Answer from the drawing. Dimensions are ordinates in mm from the lowest x, y and z of the part. A direction names the side the tool comes from. Give positions to 0.01 mm unless a question says otherwise; leave off trailing zeros. Loops run counter-clockwise (first coordinate to the right, second up) from the corner with the lowest first, then second, coordinate; pieces in that order, holes last. Notation, with made-up numbers: (-25.75, 61.5) - (-0.75, 61.5) arc R14 cw to (-0.75, 78.5) - close; hole circle Ø10 at (7, 29.5). An arc over 180 degrees is marked (long way). One line per item, written item: value.
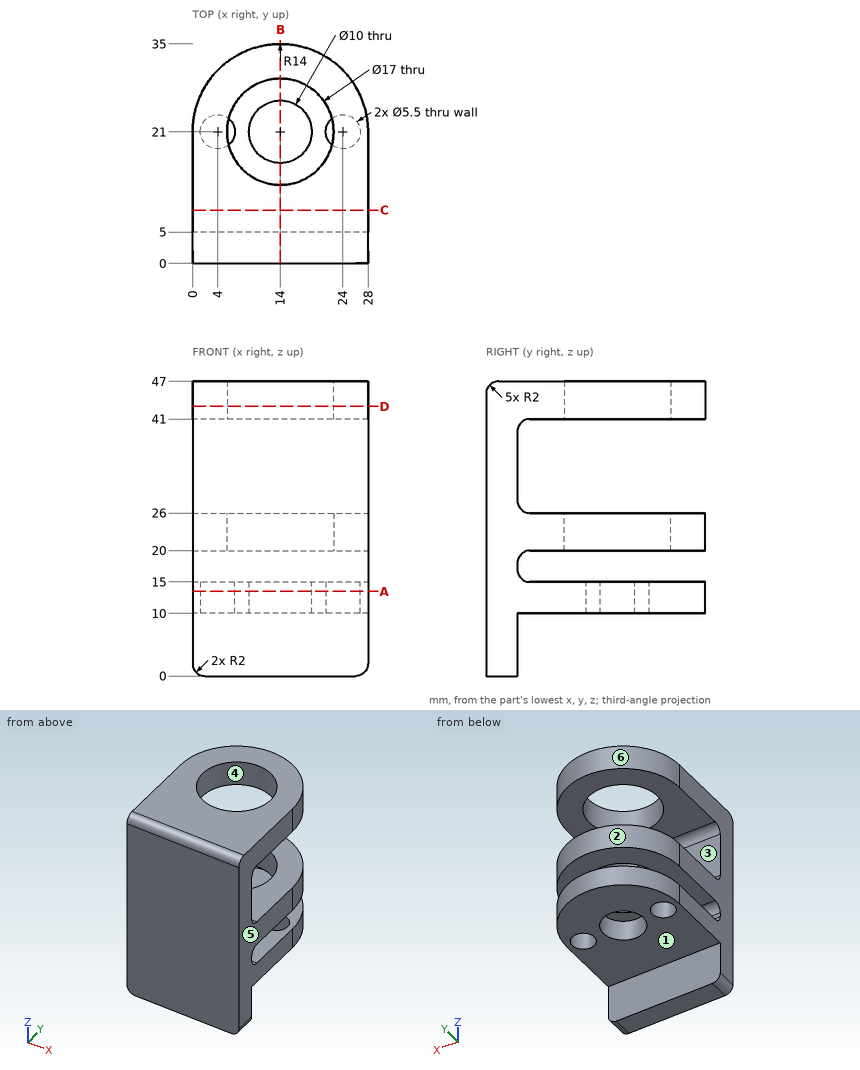
1. Section A-A (z = 13.5) is taken. Write down the section's boundary in (x, y).
Output:
outline: (0, 0) - (28, 0) - (28, 21) arc R14 ccw to (0, 21) - close; hole circle Ø5.5 at (4, 21); hole circle Ø10 at (14, 21); hole circle Ø5.5 at (24, 21)
2. Find the intervals of material crossed by line 1 along Z through (x, y) = (3, 13); line 2 along Y through (x, z) = (14, 22.6); line 3 along Y through (x, z) = (23.75, 37), in increasing order.
Output:
line 1: z = 10 to 15, 20 to 26, 41 to 47
line 2: y = 0 to 12.5, 29.5 to 35
line 3: y = 0 to 5
3. Section C-C (y = 8.5) is taken. Write down the section's boundary in (x, z).
Output:
outline: (0, 10) - (28, 10) - (28, 15) - (0, 15) - close; (0, 20) - (28, 20) - (28, 26) - (0, 26) - close; (0, 41) - (28, 41) - (28, 47) - (0, 47) - close
4. The mould has two halves that part along X. Classify the marked faces 4, 5 and 6: released by +X, released by -X, zero draft, split by the parting line, or undercut.
Output:
face 4: undercut
face 5: released by +X
face 6: split by the parting line
5. Flat-ended cylindrical pins translate along their axes: pin 1 Ø2 at (x, z) = (19, 35.5) entering from -Y; pin 2 Ø4 at (x, y) = (19.5, 22) entering from +Z; pin 3 Ø5 at (x, z) = (12.5, 5.5) entering from +Y; pin 4 Ø8.5 at (x, y) = (18.5, 21.5) entering from -Z. Find the tip coordinate at first contact, or state that the pin passes through.
Output:
pin 1: stops at y = 0
pin 2: stops at z = 15
pin 3: stops at y = 5
pin 4: stops at z = 10
6. Section B-B (x = 14) is taken. Count the separate pieces of the cut face and the enclosed holes in it, and give its area (3 significant figures).
Output:
separate pieces: 4
enclosed holes: 0
area: 494 mm²
7. For the marked faces 1, 2 and 3, determine the directions among +Z, -Z, +X, -X, +Y, -Y from which every point of the face is accessible in a straight line to the end or side of a thin tool.
Output:
face 1: -Z, +X, -X, +Y
face 2: +Z, -Z, +Y
face 3: +X, -X, +Y
8. Section D-D (z = 43) is taken. Write down the section's boundary in (x, y), and give its area (3 significant figures).
Output:
outline: (0, 0) - (28, 0) - (28, 21) arc R14 ccw to (0, 21) - close; hole circle Ø17 at (14, 21)
area: 669 mm²
